from build123d import *

# Parameters (mm, degrees)
CYLINDER028_R           = 1.6
CYLINDER028_DEPTH       = 10
CYLINDER028_PITCH_ANGLE = 90
BOX003_W                = 3
BOX003_H                = 85
BOX003_DEPTH            = 30


with BuildPart() as back_hole:
    # Cylinder028 → Cylinder028 (new body)
    with BuildSketch(Plane.XY):
        Circle(CYLINDER028_R)
    extrude(amount=CYLINDER028_DEPTH)


with BuildPart() as back_hole_1:
    # Cylinder028 pitch: moved
    add(back_hole.part.rotate(Axis((0, 0, 0), (0, 1, 0)), CYLINDER028_PITCH_ANGLE))


with BuildPart() as back_hole_2:
    # Cylinder028 placement: moved
    add(back_hole_1.part.moved(Location((97.6, 47.69, -18.9))))


with BuildPart() as final_back:
    # Box003 → Box003 (new body)
    with BuildSketch(Plane(origin=(100, 0, -25), x_dir=(1, 0, 0), z_dir=(0, 0, 1))):
        with Locations((1.5, 42.5)):
            Rectangle(BOX003_W, BOX003_H)
    extrude(amount=BOX003_DEPTH)

    # Cut025: cut back hole
    add(back_hole_2.part, mode=Mode.SUBTRACT)


solid = final_back.part
Read the model definition and answer for the solid it produces. Units are mm, in the model's axes. Round coordinates to 2 decimals unless told otherwise and drop trailing zeros. Loops run counter-clockwise (first coordinate to the right, second up) from the corner with the lowest first, then second, coordinate; pieces in that order, holes last.
Q1. Consider probe 1 along Y at (x, z) = (102.3, -18.9); probe 2 along Z at (x, y) = (101, 47.69); probe 3 along Y at (x, z) = (102.6, -19.5). Determine where each line is inside the solid, lowest interval first.
Q2. This flat-tipped pin is pushed along its axis until it touches: pin 1 (1.9 mm diameter, centred on y = 47.69, z = -18.9, fed in from -X). Where does it stop, or does it pass through?
Q3. Section B-B on y = 47.69 is taken. Write down the section's boundary in (x, z).
Q4. Determine the mould class of faces 1 (the face through (101, 85, -10)), 2 (the face through (101.48, 46.27, -19.64)), 3 (the face through (101, 43, -25)), 4 (the face through (101, 0, -10)) for opening direction Y: released by +Y, released by -Y, zero draft, split by the parting line, or undercut.
Q5. Section A-A on z = -18.9 is taken. Write down the section's boundary in (x, y).
Output:
1. probe 1: y = 0 to 46.09, 49.29 to 85
1. probe 2: z = -25 to -20.5, -17.3 to 5
1. probe 3: y = 0 to 46.21, 49.17 to 85
2. pin 1: passes through
3. outline: (100, -25) - (103, -25) - (103, -20.5) - (100, -20.5) - close; (100, -17.3) - (103, -17.3) - (103, 5) - (100, 5) - close
4. face 1: released by +Y
4. face 2: undercut
4. face 3: zero draft
4. face 4: released by -Y
5. outline: (100, 0) - (103, 0) - (103, 46.09) - (100, 46.09) - close; (100, 49.29) - (103, 49.29) - (103, 85) - (100, 85) - close
